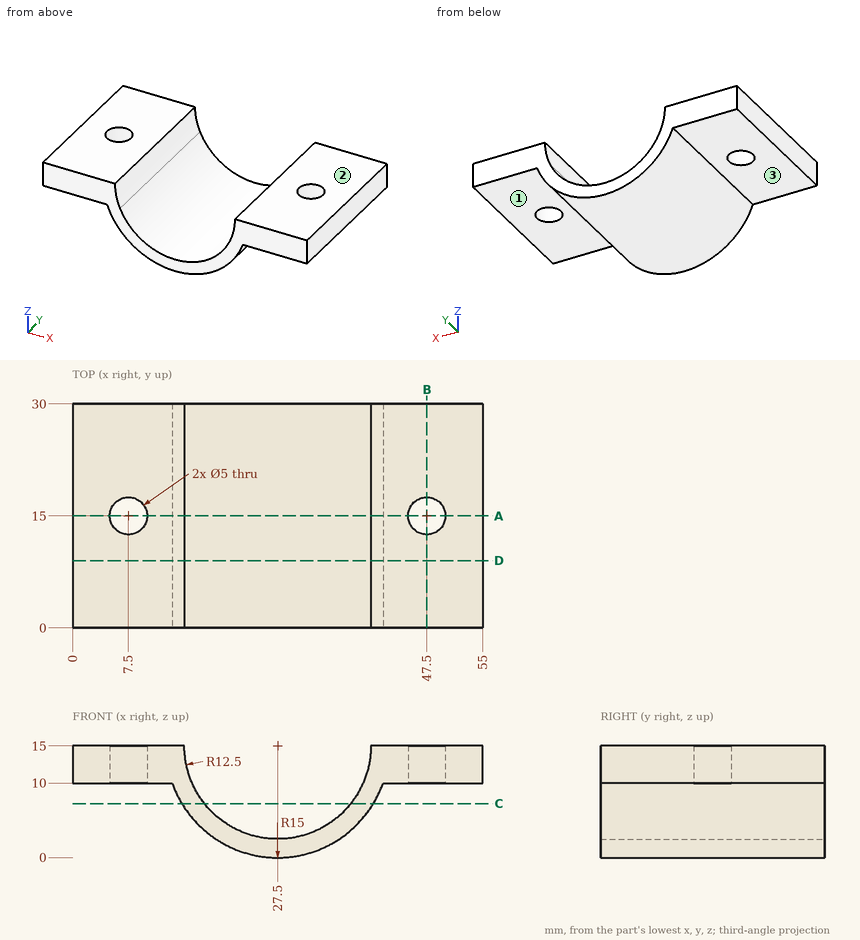
The figure shows three views and two pictorial views of one solid part (mm, origin at its lowest corner). Answer the questions. A direction names the side the tool comes from. Give positions to 0.01 mm unless a question says otherwise; leave off trailing zeros. Loops run counter-clockwise (first coordinate to the right, second up) from the corner with the lowest first, then second, coordinate; pieces in that order, holes last. Notation, with made-up numbers: (-28.75, 55) - (2.25, 55) arc R11 cw to (2.25, 66) - close; hole circle Ø10 at (51, -10). An arc over 180 degrees is marked (long way). Use one line per item in the form item = value.
1. Section C-C on z = 7.25 is taken. Give the vertices of the cut face in (x, y).
Calculated:
outline = (14.66, 0) - (17.69, 0) - (17.69, 30) - (14.66, 30) - close; (37.31, 0) - (40.34, 0) - (40.34, 30) - (37.31, 30) - close
2. Section B-B on x = 47.5 is taken. Give the vertices of the cut face in (y, z), then the cut area to 3 significant figures.
Calculated:
outline = (0, 10) - (12.5, 10) - (12.5, 15) - (0, 15) - close; (17.5, 10) - (30, 10) - (30, 15) - (17.5, 15) - close
area = 125 mm^2
3. Section A-A on y = 15 is taken. Give the vertices of the cut face in (x, z).
Calculated:
outline = (0, 10) - (5, 10) - (5, 15) - (0, 15) - close; (10, 10) - (13.36, 10) arc R15 ccw to (41.64, 10) - (45, 10) - (45, 15) - (40, 15) arc R12.5 cw to (15, 15) - (10, 15) - close; (50, 10) - (55, 10) - (55, 15) - (50, 15) - close
4. Which of the six approach directions +Z, -Z, +X, -X, +Y, -Y give full straight-line access (tool end or side, diameter ignored) to the marked faces 1, 2 and 3?
Calculated:
face_1 = -Z, +X, +Y, -Y
face_2 = +Z, +X, -X, +Y, -Y
face_3 = -Z, -X, +Y, -Y
5. Find the intervals of material crossed by line 1 along Y through (x, z) = (7.5, 12.9); line 2 along X through (y, z) = (14.5, 13.5); line 3 along X through (y, z) = (23.75, 7.5), in increasing order. Write a range as [from, to].
Calculated:
line_1 = [0, 12.5], [17.5, 30]
line_2 = [0, 5.05], [9.95, 15.09], [39.91, 45.05], [49.95, 55]
line_3 = [14.51, 17.5], [37.5, 40.49]
6. Given pin 1 Ø3 at (y, z) = (22, 2) entering from -X; pin 2 Ø12 at (x, y) = (46, 14) entering from -Z; pin 3 Ø1 at (x, y) = (19, 8) entering from -Z, each flat-ended and moving along its own axis, determine where each tip first touches the part or whether it passes through.
Calculated:
pin_1 = 17.87
pin_2 = 6.71
pin_3 = 2.31
7. Section D-D on y = 9 is taken. Give the vertices of the cut face in (x, z).
Calculated:
outline = (0, 10) - (13.36, 10) arc R15 ccw to (41.64, 10) - (55, 10) - (55, 15) - (40, 15) arc R12.5 cw to (15, 15) - (0, 15) - close
